CAD build for the part. Positions are in the model's coordinates, mm. Face numbers are marked on the shaded views. A direction names the side the tool comes from. Round coordinates to 2 decimals unless told otherwise and drop trailing zeros. Order: outer loops, then holes, each group sorted by start corner. A loop starts at its lowest first (then second) coordinate and runs counter-clockwise, first axis right, second up. Notation, with made-up numbers: (-5.5, -5.75) -> (2.5, -5.75) arc R9 cw to (2.5, 6.25) -> close; hole circle Ø11 at (65, 50). An arc over 180 degrees is marked (long way). Return JSON: item names as keys, results as strings. Group by question number.
Q1. Probe line 1 along X through (y, z) = (-3, -5.75); line 2 along X through (y, z) = (-1.5, -7.5); line 3 along Z through (x, y) = (-0.3, 4.5). List the from-to ranges inside material, lowest first.
Q2. Mould opens along X. For the marked faces 3, 4 and 5 say: +X half, -X half, draft (parallel to the pull), parting line (faces both ways), or undercut.
Q3. Cut at C-C (z = -1.5). Write the cut outline in (x, y), then the cut area to 3 significant figures.
Q4. Which spindle directions (+Z, -Z, +X, -X, +Y, -Y) get a long thin tool onto all of the face, cutting with end or side? Do the marked faces 1 and 2. Say none if no direction does.
Q5. Cut at A-A (z = -3.5). Write the cut outline in (x, y).
Q6. Cut at B-B (x = -0.2). Write the cut outline in (y, z).
Q7. Flat gauge pin, fed straight in: pin 1 (1 mm diameter, centred on x = -0.5, y = -4, fed in from +Z). Where does the tip first touch, or does it go through?
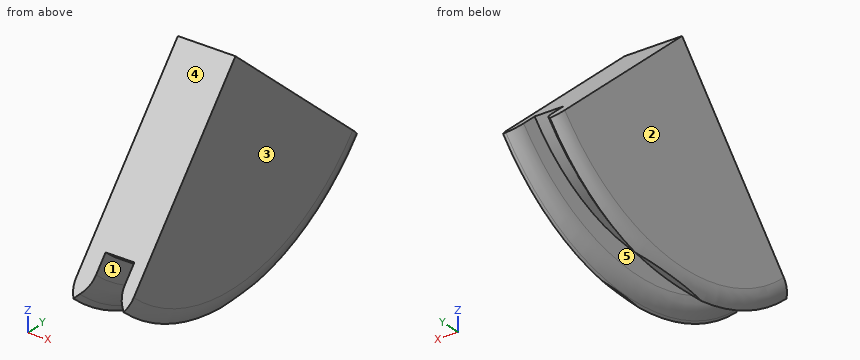
from build123d import *

# Parameters (mm, degrees)
CUT_EXTRUDE1_DEPTH      = 12.33524834
CUT_EXTRUDE1_DEPTH_BACK = 12.33524834
SKETCH3_OUTSIDE_W       = 22.502
SKETCH3_OUTSIDE_H       = 22.502


with BuildPart() as part:
    # Sketch2 → Revolve1 (revolve)
    with BuildSketch(Plane(origin=(0, 0, 0), x_dir=(1, 0, 0), z_dir=(0, 1, 0)), mode=Mode.PRIVATE) as revolve1_sk:
        with BuildLine():
            Line((-1, 0), (1, 0))
            Line((1, 0), (1, 5.5))
            Line((1, 5.5), (1, 7.395254938))
            ThreePointArc((1, 7.395254938), (0.968908672, 7.642673583), (0.877568029, 7.874707079))
            add(Edge.make_bspline(
                [(0.820511391, 7.803982399), (0.850646042, 7.838050546), (0.877568029, 7.874707079)],
                knots=[2.4177114, 2.4177114, 2.4177114, 2.508439234, 2.508439234, 2.508439234], degree=2, weights=[1, 0.998971234, 1]))
            ThreePointArc((0.820511391, 7.803982399), (0.634382255, 7.495682579), (0.569535838, 7.14144004))
            Line((0.569535838, 7.14144004), (0.569535838, 6.447627469))
            Line((0.569535838, 6.447627469), (-0.430464162, 6.447627469))
            Line((-0.430464162, 6.447627469), (-0.430464162, 7.14144004))
            ThreePointArc((-0.430464162, 7.14144004), (-0.495310579, 7.495682579), (-0.681439715, 7.803982399))
            add(Edge.make_bspline(
                [(-0.80833384, 7.983979325), (-0.754845236, 7.886969591), (-0.681439715, 7.803982399)],
                knots=[0.503618874, 0.503618874, 0.503618874, 0.723881254, 0.723881254, 0.723881254], degree=2, weights=[1, 0.993941688, 1]))
            ThreePointArc((-0.80833384, 7.983979325), (-0.950876921, 7.704824123), (-1, 7.395254938))
            Line((-1, 7.395254938), (-1, 5.5))
            Line((-1, 5.5), (-1, 0))
        make_face()
    revolve(revolve1_sk.sketch.rotate(Axis((0, 0, 0), (1, 0, 0)), 180), axis=Axis((0, 0, 0), (1, 0, 0)))

    # Sketch3 outside → Cut-Extrude1 (cut, two sides: drawn at the far end of the back side and taken through both)
    with BuildSketch(Plane(origin=(0, 0, 0), x_dir=(0, 0, -1), z_dir=(1, 0, 0)).offset(-CUT_EXTRUDE1_DEPTH_BACK)):
        Rectangle(SKETCH3_OUTSIDE_W, SKETCH3_OUTSIDE_H)
        Polygon((0, 0), (7.412882699, 8.555619308), (8.184858407, -7.091642708), align=None, mode=Mode.SUBTRACT)
    extrude(amount=CUT_EXTRUDE1_DEPTH + CUT_EXTRUDE1_DEPTH_BACK, mode=Mode.SUBTRACT)


solid = part.part
Solution:
{
 "1": {"line 1": "x = -1 to -0.43, 0.57 to 1", "line 2": "x = -0.97 to -0.57, 0.71 to 0.97", "line 3": "z = -4.62 to -3.9"},
 "2": {"face 3": "+X half", "face 4": "draft", "face 5": "undercut"},
 "3": {"outline": "(-1, -1.3) -> (1, -1.3) -> (1, 1.73) -> (-1, 1.73) -> close", "area": "6.06 mm²"},
 "4": {"face 1": "-Z", "face 2": "+Z, -Z, -X, +Y, -Y"},
 "5": {"outline": "(-1, -3.03) -> (1, -3.03) -> (1, 4.04) -> (-1, 4.04) -> close"},
 "6": {"outline": "(-4.22, -4.87) arc R6.45 ccw to (4.87, -4.22) -> (0, 0) -> close"},
 "7": {"pin 1": "stops at z = -4.04"}
}
